Here's how the part is built. I have some questions about the finished solid (model axes, mm). A direction names the side the tool comes from. Round coordinates to 2 decimals unless told otherwise and drop trailing zeros. Write each loop counter-clockwise with the first axis right and the second up, starting at its lowest first coordinate (ties: lowest second). Pieces come first, ordered by that corner, then holes. Notation, with made-up numbers: (-38.75, 6) - (-26.75, 6) arc R19 ccw to (-26.75, 15) - close; hole circle Ø6 at (70.25, 73.25). An arc over 180 degrees is marked (long way). Return JSON: item names as keys, results as strings. Group by question number.
```python
from build123d import *

# Parameters (mm, degrees)
T_LE_DE_BASE_PLI_E1_DEPTH = 226
CONG_1_R                  = 15
ESQUISSE2_W               = 270.5
ESQUISSE2_H               = 65.5
ENL_V_MAT_EXTRU_1_DEPTH   = 80
ESQUISSE6_W               = 0.5
ESQUISSE6_H               = 30
ENL_V_MAT_EXTRU_2_DEPTH   = 10


# Read off the part's stored shape, not the designer's step: Tôle de base pliée1
with BuildPart() as part:
    # Tôle de base pliée1 outline → Tôle de base pliée1 (new body)
    with BuildSketch(Plane(origin=(0, 0, 0), x_dir=(1, 0, 0), z_dir=(0, 1, 0))):
        with BuildLine():
            Line((-219.5, 85), (-219.5, 29))
            Line((-219.5, 29), (-218.5, 29))
            Line((-218.5, 29), (-218.5, 85))
            ThreePointArc((-218.5, 85), (-216.01040764, 91.01040764), (-210, 93.5))
            Line((-210, 93.5), (210, 93.5))
            ThreePointArc((210, 93.5), (216.01040764, 91.01040764), (218.5, 85))
            Line((218.5, 85), (218.5, -40))
            ThreePointArc((218.5, -40), (216.01040764, -46.01040764), (210, -48.5))
            Line((210, -48.5), (131.5, -48.5))
            Line((131.5, -48.5), (131.5, -49.5))
            Line((131.5, -49.5), (210, -49.5))
            ThreePointArc((210, -49.5), (216.717514421, -46.717514421), (219.5, -40))
            Line((219.5, -40), (219.5, 85))
            ThreePointArc((219.5, 85), (216.717514421, 91.717514421), (210, 94.5))
            Line((210, 94.5), (-210, 94.5))
            ThreePointArc((-210, 94.5), (-216.717514421, 91.717514421), (-219.5, 85))
        make_face()
    extrude(amount=T_LE_DE_BASE_PLI_E1_DEPTH)

    # Congé1
    cong_1_edges = [part.edges().sort_by_distance(p)[0] for p in [
        (131.5, 226, 49),
    ]]
    fillet(cong_1_edges, radius=CONG_1_R)

    # Esquisse2 → Enlèv. mat.-Extru.1 (cut)
    with BuildSketch(Plane(origin=(0, 226, 0), x_dir=(1, 0, 0), z_dir=(0, 1, 0))):
        with Locations((-84.25, 61.75)):
            Rectangle(ESQUISSE2_W, ESQUISSE2_H)
    extrude(amount=-ENL_V_MAT_EXTRU_1_DEPTH, mode=Mode.SUBTRACT)

    # Esquisse6 → Enlèv. mat.-Extru.2 (cut)
    with BuildSketch(Plane(origin=(0, 0, -94.5), x_dir=(-1, 0, 0), z_dir=(0, 0, -1))):
        with Locations((120, 131)):
            Rectangle(ESQUISSE6_W, ESQUISSE6_H)
        with Locations((150, 131)):
            Rectangle(ESQUISSE6_W, ESQUISSE6_H)
    extrude(amount=-ENL_V_MAT_EXTRU_2_DEPTH, mode=Mode.SUBTRACT)


solid = part.part
```
1) If we mould it in two halves opening along X, with no side actions, what happens to faces 1 (the flat face through (-219.5, 72, -57)), 2 (the cylindrical face through (216.643, 111.418, 46.791)), 3 (the cylindrical face through (-216.08, 71.98, -90.94))? For each: released by +X, released by -X, zero draft, split by the parting line, or undercut.
2) Imagine slicing it at D-D (x = -111). Please give me the cut outline in (y, z).
3) Imagine slicing it at C-C (y = 167). Please give me the cut outline in (x, z), plus the area to 3 significant figures.
4) I need wall thicknesses on line 1 along X through (y, z) = (73, -70); line 2 along Z through (x, y) = (200.5, 25.5); line 3 along Z through (x, y) = (108, 23). Which ranges of each line are inside material? Lowest first, please.
5) For faces 4 (the cylindrical face through (216.08, 111.42, 45.94)), 5 (the flat face through (-218.5, 72, -57)), 6 (the cylindrical face through (215.94, 111.42, -91.08)), which set-ups out of +Z, -Z, +X, -X, +Y, -Y let a thin tool reach every point of the face, with its end or its side?
6) Imagine slicing it at B-B (z = -74). Please give me the cut outline in (x, y).
7) Imagine slicing it at A-A (x = 172.5). Please give me the cut outline in (y, z).
8) Will these pins go through, and if not, where does the flat tip stop? pin 1 Ø1.1 at (y, z) = (187.5, -94) entering from -X; pin 2 Ø1.1 at (y, z) = (126.5, -94) entering from +X; pin 3 Ø1.1 at (x, z) = (-64.5, -94) entering from +Y.
Results found:
{
 "1": {"face 1": "released by -X", "face 2": "released by +X", "face 3": "undercut"},
 "2": {"outline": "(0, -94.5) - (146, -94.5) - (146, -93.5) - (0, -93.5) - close"},
 "3": {"outline": "(51, -94.5) - (210, -94.5) arc R9.5 ccw to (219.5, -85) - (219.5, 40) arc R9.5 ccw to (210, 49.5) - (131.5, 49.5) - (131.5, 48.5) - (210, 48.5) arc R8.5 cw to (218.5, 40) - (218.5, -85) arc R8.5 cw to (210, -93.5) - (51, -93.5) - close", "area": "391 mm²"},
 "4": {"line 1": "x = -219.5 to -218.5, 218.5 to 219.5", "line 2": "z = -94.5 to -93.5, 48.5 to 49.5", "line 3": "z = -94.5 to -93.5"},
 "5": {"face 4": "-X, +Y, -Y", "face 5": "+Z, +Y, -Y", "face 6": "+Y, -Y"},
 "6": {"outline": "(-219.5, 0) - (-218.5, 0) - (-218.5, 146) - (-219.5, 146) - close; (218.5, 0) - (219.5, 0) - (219.5, 226) - (218.5, 226) - close"},
 "7": {"outline": "(0, -94.5) - (226, -94.5) - (226, -93.5) - (0, -93.5) - close; (0, 48.5) - (226, 48.5) - (226, 49.5) - (0, 49.5) - close"},
 "8": {"pin 1": "stops at x = 51", "pin 2": "stops at x = 214.34", "pin 3": "stops at y = 146"}
}
